Read the model definition and answer for the solid it produces. Units are mm, in the model's axes. A direction names the side the tool comes from. Coordinates: 2 decimals unless noted, no trailing zeros. Write each loop counter-clockwise with the first axis right and the second up, starting at its lowest first coordinate (ties: lowest second). Pieces come first, ordered by that corner, then holes.
Item 1: Each of these flat-tipped pins is pushed along its axis until it touches: P1, Ø0.6, axis at x = -3, z = 8.5, coming from the +Y side; P2, Ø1, axis at y = -26.5, z = 7.5, coming from the -X side; P3, Ø5, axis at y = -9, z = 2, coming from the -X side; P4, Ø1.5, axis at x = 6.5, y = 17.5, coming from the +Z side. Where does it stop, or does it pass through?
Item 2: Determine the mould class of faces 6 (the face through (-22.74, 16.61, 6.08)), 7 (the face through (-26.184, -14.642, 5.916)), 8 (the face through (0, 30, 6)), 9 (the face through (-21.39, 16.97, 6.08)) for opening direction Y: released by +Y, released by -Y, zero draft, split by the parting line, or undercut.
Item 3: Straight lines are drawn through the part: probe 1 along Y at (x, z) = (-0.5, 6.25); probe 2 along X at (y, z) = (-4, 4.75); probe 3 along Y at (x, z) = (-7.5, 2.5). For each, find the intervals that lie inside material, in ascending order.
Item 4: Section C-C (y = -12.5) is taken. Give the vertices of the cut face in (x, z), then the cut area to 3 significant figures.
Item 5: Section A-A (x = 0) is taken. Give the vertices of the cut face in (y, z).
Item 6: Section D-D (z = 1.25) is taken. Give the vertices of the cut face in (x, y), then the cut area to 3 significant figures.
Item 7: A tool of negligible diameter and unlimited length cuts with its end or side. For faces 1 (the face through (25.39, 10.04, 6.08)), 2 (the face through (-2, -29, 6)), 3 (the face through (0, -6, 0)), 4 (the face through (24.098, 16.222, 6.084)), 5 (the face through (-26.1, 12.76, 6.08)), from which of +Z, -Z, +X, -X, +Y, -Y can it reach the whole face along a straight path? Write none if from no direction.
Item 8: Section B-B (x = -15) is taken. Give the vertices of the cut face in (y, z), then the cut area to 3 significant figures.
from build123d import *

# Parameters (mm, degrees)
SKETCH_R              = 30
PAD_DEPTH             = 12
SKETCH001_R           = 9.2
POCKET_DEPTH          = 183.395282
POLARPATTERN_COUNT    = 3
SKETCH002_R           = 1.8
POCKET001_DEPTH       = 12.001
SKETCH003_W           = 4
SKETCH003_H           = 4
SKETCH003_W_2         = 8
SKETCH003_H_2         = 2
POCKET002_DEPTH       = 183.395282
POLARPATTERN001_COUNT = 3


with BuildPart() as part:
    # Sketch → Pad (new body)
    with BuildSketch(Plane.XY):
        Circle(SKETCH_R)
    extrude(amount=PAD_DEPTH)

    # Sketch001 (on Face3 of Pad) → Pocket (cut, through all)
    with BuildSketch(Plane.XY.offset(12)):
        with Locations((0, 13)):
            Circle(SKETCH001_R)
    pocket = extrude(amount=-POCKET_DEPTH, mode=Mode.SUBTRACT)

    # PolarPattern: Pocket ×3 about axis
    polarpattern_axis = Axis((0, 0, 12), (0, 0, 1))
    for i in range(1, POLARPATTERN_COUNT):
        add(pocket.rotate(polarpattern_axis, i * 360 / POLARPATTERN_COUNT), mode=Mode.SUBTRACT)

    # Sketch002 (on Face3 of PolarPattern) → Pocket001 (cut, through all)
    with BuildSketch(Plane.XY.offset(12)):
        Circle(SKETCH002_R)
    extrude(amount=-POCKET001_DEPTH, mode=Mode.SUBTRACT)

    # Sketch003 (on Face3 of Pocket001) → Pocket002 (cut, through all)
    with BuildSketch(Plane.XY.offset(12)):
        with Locations((0, -30)):
            Rectangle(SKETCH003_W, SKETCH003_H)
        with Locations((0, -27)):
            Rectangle(SKETCH003_W_2, SKETCH003_H_2)
    pocket002 = extrude(amount=-POCKET002_DEPTH, mode=Mode.SUBTRACT)

    # PolarPattern001: Pocket002 ×3 about axis
    polarpattern001_axis = Axis((0, 0, 12), (0, 0, 1))
    for i in range(1, POLARPATTERN001_COUNT):
        add(pocket002.rotate(polarpattern001_axis, i * 360 / POLARPATTERN001_COUNT), mode=Mode.SUBTRACT)


solid = part.part
Established:
1. P1: stops at y = 29.88
1. P2: stops at x = -14.97
1. P3: stops at x = -29.29
1. P4: passes through
2. face 6: undercut
2. face 7: split by the parting line
2. face 8: released by +Y
2. face 9: undercut
3. probe 1: y = -26 to -1.73, 1.73 to 3.81, 22.19 to 30
3. probe 2: x = -29.73 to -20.11, -2.4 to 2.4, 20.11 to 29.73
3. probe 3: y = -29.05 to -14.9, 1.9 to 7.67, 18.33 to 29.05
4. outline: (-27.27, 0) - (-18.23, 0) - (-18.23, 12) - (-27.27, 12) - close; (-4.28, 0) - (4.28, 0) - (4.28, 12) - (-4.28, 12) - close; (18.23, 0) - (27.27, 0) - (27.27, 12) - (18.23, 12) - close
4. area: 320 mm2
5. outline: (-26, 0) - (-1.8, 0) - (-1.8, 12) - (-26, 12) - close; (1.8, 0) - (3.8, 0) - (3.8, 12) - (1.8, 12) - close; (22.2, 0) - (30, 0) - (30, 12) - (22.2, 12) - close
6. outline: (-26.92, 13.23) arc R30 ccw to (-2, -29.93) - (-2, -28) - (-4, -28) - (-4, -26) - (4, -26) - (4, -28) - (2, -28) - (2, -29.93) arc R30 ccw to (26.92, 13.23) - (25.25, 12.27) - (26.25, 10.54) - (24.52, 9.54) - (20.52, 16.46) - (22.25, 17.46) - (23.25, 15.73) - (24.92, 16.7) arc R30 ccw to (-24.92, 16.7) - (-23.25, 15.73) - (-22.25, 17.46) - (-20.52, 16.46) - (-24.52, 9.54) - (-26.25, 10.54) - (-25.25, 12.27) - close; hole circle Ø18.4 at (-11.26, -6.5); hole circle Ø18.4 at (0, 13); hole circle Ø3.6 at (0, 0); hole circle Ø18.4 at (11.26, -6.5)
6. area: 1,950 mm2
7. face 1: +Z, -Z
7. face 2: +Z, -Z, -Y
7. face 3: -Z, +X, -X, +Y, -Y
7. face 4: +Z, -Z, +X
7. face 5: +Z, -Z, +Y
8. outline: (-25.98, 0) - (-14.9, 0) - (-14.9, 12) - (-25.98, 12) - close; (1.9, 0) - (25.98, 0) - (25.98, 12) - (1.9, 12) - close
8. area: 422 mm2
